```python
from build123d import *

# Parameters (mm, degrees)
SKETCH_1_R      = 6
SKETCH_1_R_2    = 1.5
EXTRUDE_1_DEPTH = 3
FILLET_2_R      = 1
FILLET_3_R      = 1


with BuildPart() as part:
    # 草图1 → 凸台-拉伸1 (new body)
    with BuildSketch(Plane.XY):
        Circle(SKETCH_1_R)
        Circle(SKETCH_1_R_2, mode=Mode.SUBTRACT)
    extrude(amount=EXTRUDE_1_DEPTH)

    # 圆角2
    fillet_2_edges = [part.edges().sort_by_distance(p)[0] for p in [
        (-6, 0, 0),
    ]]
    fillet(fillet_2_edges, radius=FILLET_2_R)

    # 圆角3
    fillet_3_edges = [part.edges().sort_by_distance(p)[0] for p in [
        (-6, 0, 3),
        (-1.5, 0, 3),
    ]]
    fillet(fillet_3_edges, radius=FILLET_3_R)


solid = part.part
```
Geometry check sheet. Reference: the model listing, model coordinates, mm. Give positions to 0.01 mm unless a question says otherwise; leave off trailing zeros. Order: outer loops, then holes, each group sorted by start corner. A loop starts at its lowest first (then second) coordinate and runs counter-clockwise, first axis right, second up.
1. Gauge pin test, flat ends, axial feed: pin 1 Ø3.5 at (x, y) = (0, 0) entering from +Z; pin 2 Ø1 at (y, z) = (4, 1) entering from -X. Record the tip position at first contact, or that the pin passes through.
2. Section check C-C, the plane z = 1.85. Enter the section's corners in (x, y).
3. Section check A-A, the plane x = 0. Enter the section's corners in (y, z), and give its area (3 significant figures).
4. Thickness scan on L1, parallel to Y at x = 0, z = 1; L2, parallel to X at y = 0.25, z = 1.4; L3, parallel to Y at x = 1.25, z = 0.65. Record the ranges inside material, lowest first.
5. Section check D-D, the plane z = 2.7. Enter the section's corners in (x, y).
6. Release check for a two-part mould opening along Y. For faces 1 (the face through (2, -2, 3)), 2 (the face through (-5.994, 0.264, 1.493)), 3 (the face through (-1.5, 0.07, 0.99)) record: pulls with the +Y half, pulls with the -Y half, needs draft (parallel to the pull), parting line crosses it, or undercut.
Values follow:
1. pin 1: stops at z = 2.66
1. pin 2: stops at x = -4.87
2. outline: circle Ø12 at (0, 0); hole circle Ø3 at (0, 0)
3. outline: (-6, 1) arc R1 ccw to (-5, 0) - (-1.5, 0) - (-1.5, 2) arc R1 ccw to (-2.5, 3) - (-5, 3) arc R1 ccw to (-6, 2) - close; (1.5, 0) - (5, 0) arc R1 ccw to (6, 1) - (6, 2) arc R1 ccw to (5, 3) - (2.5, 3) arc R1 ccw to (1.5, 2) - close
3. area: 25.7 mm2
4. L1: y = -6 to -1.5, 1.5 to 6
4. L2: x = -5.99 to -1.48, 1.48 to 5.99
4. L3: y = -5.8 to -0.83, 0.83 to 5.8
5. outline: circle Ø11.43 at (0, 0); hole circle Ø3.57 at (0, 0)
6. face 1: needs draft
6. face 2: parting line crosses it
6. face 3: undercut
